Geometry: final body of the model. Coordinates: model frame, mm. A direction names the side the tool comes from. Give positions to 0.01 mm unless a question says otherwise; leave off trailing zeros. Order: outer loops, then holes, each group sorted by start corner. A loop starts at its lowest first (then second) coordinate and runs counter-clockwise, first axis right, second up. Notation, with made-up numbers: (23.5, -38.75) - (54.5, -38.75) arc R14 ccw to (54.5, -16.75) - close; hole circle Ø7 at (33, 48). An arc over 180 degrees is marked (long way). Use one line per item in the form item = value.
Autodesk Inventor part; units mm, degrees
ref_plane "YZ Plane" through (0, 0, 0) normal (1, 0, 0) x (0, 1, 0)
ref_plane "XZ Plane" through (0, 0, 0) normal (0, 1, 0) x (-1, 0, 0)
ref_plane "XY Plane" through (0, 0, 0) normal (0, 0, 1) x (1, 0, 0)
sketch "Sketch1" plane through (0, 0, 0) normal (0, 1, 0) x (-1, 0, 0)
  line L0 (-40.2798, 52.2721) -> (31.3202, 52.2721)
  line L1 (-40.2798, 15.7721) -> (-40.2798, 52.2721)
  line L2 (-55.2966, 15.7721) -> (-40.2798, 15.7721)
  line L3 (-56.9798, 14.0889) -> (-56.9798, -48.5447)
  line L4 (46.337, -50.2279) -> (-55.2966, -50.2279)
  line L5 (48.0202, -24.2779) -> (48.0202, -48.5447)
  line L6 (48.0202, -9.7779) -> (48.0202, 14.0889)
  line L7 (31.3202, 15.7721) -> (46.337, 15.7721)
  line L8 (31.3202, 15.7721) -> (31.3202, 52.2721)
  line L9 (-56.784, 14.6914) -> (-56.9798, 14.0889)
  line L10 (-56.784, 14.6914) -> (-56.4116, 15.2039)
  line L11 (-55.2966, 15.7721) -> (-55.8991, 15.5763)
  line L12 (-56.4116, 15.2039) -> (-55.8991, 15.5763)
  spline S0 degree 4 poles (-56.9798, 14.0889) (-56.8811, 14.7163) (-56.5148, 15.3071) (-55.924, 15.6734) (-55.2966, 15.7721) knots 0 0 0 0 0 1 1 1 1 1
  line L13 (47.8244, 14.6914) -> (47.452, 15.2039)
  line L14 (46.337, 15.7721) -> (46.9395, 15.5763)
  line L15 (47.8244, 14.6914) -> (48.0202, 14.0889)
  line L16 (46.9395, 15.5763) -> (47.452, 15.2039)
  spline S1 degree 4 poles (46.337, 15.7721) (46.9644, 15.6734) (47.5552, 15.3071) (47.9215, 14.7163) (48.0202, 14.0889) knots 0 0 0 0 0 1 1 1 1 1
  line L17 (46.337, -50.2279) -> (46.9395, -50.0321)
  line L18 (47.452, -49.6597) -> (47.8244, -49.1472)
  line L19 (47.452, -49.6597) -> (46.9395, -50.0321)
  spline S2 degree 4 poles (48.0202, -48.5447) (47.9214, -49.1721) (47.5553, -49.763) (46.9644, -50.1292) (46.337, -50.2279) knots 0 0 0 0 0 1 1 1 1 1
  line L20 (-56.9798, -48.5447) -> (-56.784, -49.1472)
  line L21 (-55.2966, -50.2279) -> (-55.8991, -50.0321)
  spline S3 degree 4 poles (-55.2966, -50.2279) (-55.924, -50.1292) (-56.5149, -49.763) (-56.8811, -49.1721) (-56.9798, -48.5447) knots 0 0 0 0 0 1 1 1 1 1
  line L22 (48.0202, -9.7779) -> (48.0202, -24.2779)
  line L23 (-55.2966, 20.7721) -> (-45.2798, 20.7721)
  line L24 (-45.2798, 20.7721) -> (-45.2798, 57.2721)
  line L25 (-45.2798, 57.2721) -> (36.3202, 57.2721)
  line L26 (36.3202, 57.2721) -> (36.3202, 20.7721)
  line L27 (46.337, -55.2279) -> (-55.2966, -55.2279)
  line L28 (-61.9798, -48.5447) -> (-61.9798, 14.8809)
  line L29 (-45.2798, 20.7721) -> (-61.9798, 20.7721)
  line L30 (-61.9798, 20.7721) -> (-61.9798, -55.2279)
  line L31 (-61.9798, -55.2279) -> (53.0202, -55.2279)
  line L32 (53.0202, -55.2279) -> (53.0202, 20.7721)
  line L33 (53.0202, 20.7721) -> (36.3202, 20.7721)
  circle A0 centre (-45.2798, 20.7721) radius 2.25
  circle A1 centre (36.3202, 20.7721) radius 2.25
  circle A2 centre (0, -55.2279) radius 2.25
  circle A3 centre (36.3202, 20.7721) radius 4
  circle A4 centre (-45.2798, 20.7721) radius 4
  circle A5 centre (0, -55.2279) radius 4
  point P0 (0, 0)
  point P1 (32.0202, -45.2279)
  point P2 (-56.4116, -49.6597)
  point P3 (-56.4116, -49.6597)
  point P4 (40.3202, 20.7721)
  point P5 (36.3202, 24.7721)
  point P6 (-45.2798, 24.7721)
  point P7 (-49.2798, 20.7721)
  point P8 (-4, -55.2279)
  point P9 (4, -55.2279)
  point P10 (-56.9798, 14.0889)
  dimension "d0" = 5
  dimension "d2" = 5
  dimension "d3" = 5
  dimension "d4" = 4.5
  dimension "d5" = 4.5
  dimension "d6" = 4.5
  dimension "d7" = 8
  dimension "d8" = 8
  dimension "d9" = 8
extrude "Extrusion1" add sketch "Sketch1" along normal blind 5 contours L23 A4 L24 L25 L26 A3 L33 L32 L31 L27 A5 L30 L28 L29 | A4 L24 A0 L23 | L23 A0 L24 A4 | A3 L33 A1 L26 | L26 A1 L33 A3 | A5 L27 A2 | L27 A2 A5
sketch "Sketch2" plane through (0, 0, 0) normal (0, -1, 0) x (1, 0, 0)
  line L0 (61.9798, 20.7721) -> (61.9798, -55.2279)
  line L1 (49.2798, 20.7721) -> (61.9798, 20.7721)
  arc A0 (49.2798, 20.7721) -> (45.2798, 24.7721) centre (45.2798, 20.7721) ccw
  line L2 (45.2798, 57.2721) -> (45.2798, 24.7721)
  line L3 (-36.3202, 57.2721) -> (45.2798, 57.2721)
  line L4 (-36.3202, 24.7721) -> (-36.3202, 57.2721)
  arc A1 (-36.3202, 24.7721) -> (-40.3202, 20.7721) centre (-36.3202, 20.7721) ccw
  line L5 (-53.0202, 20.7721) -> (-40.3202, 20.7721)
  line L6 (-53.0202, -55.2279) -> (-53.0202, 20.7721)
  line L7 (-4, -55.2279) -> (-53.0202, -55.2279)
  arc A2 (-4, -55.2279) -> (4, -55.2279) centre (0, -55.2279) ccw
  line L8 (61.9798, -55.2279) -> (4, -55.2279)
  circle A3 centre (45.2798, 20.7721) radius 2.25
  circle A4 centre (45.2798, 20.7721) radius 2.25
  circle A5 centre (0, -55.2279) radius 2.25
  circle A6 centre (-36.3202, 20.7721) radius 2.25
  point P0 (0, 0)
extrude "Extrusion2" add sketch "Sketch2" along normal blind 3
properties part number "raspberry-coral-chasis-fastening"
(1) Cut plane B-B on z = 43. Output: boundary loops of the cut face in (x, y).
Computed values:
outline = (-36.32, -3) - (45.28, -3) - (45.28, 5) - (40.28, 5) - (40.28, 0) - (-31.32, 0) - (-31.32, 5) - (-36.32, 5) - close
(2) Cut plane D-D on y = 2.5. Give the number of separate pieces and of enclosed holes in the cut face, plus the area to 3 significant figures.
Computed values:
separate_pieces = 1
enclosed_holes = 4
area = 2,180 mm²
(3) Reachability of faces 1 (the face through (56, 1, 20.772)), 2 (the face through (-48.02, 2, -17)), 3 (the face through (-28, 1, -55.228)), 4 (the face through (-47, 1, 20.772)) from +Z, -Z, +X, -X, +Y, -Y: full face, straight path, thin tool, end or side. Return the list, or none.
Computed values:
face_1 = +Z, +X, +Y, -Y
face_2 = +Y
face_3 = -Z, -X, +Y, -Y
face_4 = +Z, -X, +Y, -Y
(4) Ray query, line 1 along X through (y, z) = (2.75, 9); line 2 along X through (y, z) = (3, 48.5); line 3 along Z through (x, y) = (-32.5, 4). Return the intervals inside material, ascending.
Computed values:
line_1 = -53.02 to -48.02, 56.98 to 61.98
line_2 = -36.32 to -31.32, 40.28 to 45.28
line_3 = -55.23 to -50.23, 15.77 to 57.27
(5) Pull-direction query (X, two-part tool) for faces 5 (the face through (43, 5, 17)), 6 (the face through (-31.32, 2, 34)), 7 (the face through (-53.02, 1, -18)); classes: released by +X, released by -X, zero draft, split by the parting line, or undercut.
Computed values:
face_5 = zero draft
face_6 = undercut
face_7 = released by -X
(6) Cut plane A-A on x = 0. Output: boundary loops of the cut face in (y, z), plus the area to 4 significant figures.
Computed values:
outline = (-3, -59.23) - (5, -59.23) - (5, -57.48) - (-3, -57.48) - close; (-3, -52.98) - (5, -52.98) - (5, -50.23) - (0, -50.23) - (0, 52.27) - (5, 52.27) - (5, 57.27) - (-3, 57.27) - close
area = 383.5 mm²
(7) Contact query for flat-ended pins moving along their axis: pin 1 Ø2.5 at (x, z) = (45.28, 20.77) entering from -Y; pin 2 Ø4 at (y, z) = (-1, 36.5) entering from +X; pin 3 Ø4 at (x, y) = (-44.5, -1) entering from +Z; pin 4 Ø2.5 at (x, y) = (48.5, 1.5) entering from -Z. Output: stop coordinate, or through.
Computed values:
pin_1 = through
pin_2 = 45.28
pin_3 = 20.77
pin_4 = -55.23
(8) Cut plane C-C on x = 15. Output: boundary loops of the cut face in (y, z), plus the area to 4 significant figures.
Computed values:
outline = (-3, -55.23) - (5, -55.23) - (5, -50.23) - (0, -50.23) - (0, 52.27) - (5, 52.27) - (5, 57.27) - (-3, 57.27) - close
area = 387.5 mm²
